Source: CAD feature listing. Evaluate the final solid. Frame: model axes, mm. A direction names the side the tool comes from. Give positions to 0.01 mm unless a question says otherwise; leave off trailing zeros. Loops run counter-clockwise (first coordinate to the right, second up) from the corner with the lowest first, then second, coordinate; pieces in that order, holes last.
from build123d import *

# Parameters (mm, degrees)
SKETCH_W        = 160
SKETCH_H        = 80
PAD_DEPTH       = 32
POCKET_DEPTH    = 26
SKETCH002_R     = 6
POCKET001_DEPTH = 1
SKETCH003_R     = 6
POCKET002_DEPTH = 1
SKETCH004_R     = 3.1
POCKET003_DEPTH = 4
SKETCH005_R     = 3.1
POCKET004_DEPTH = 4
FILLET_R        = 4
FILLET001_R     = 1


with BuildPart() as part:
    # Sketch → Pad (new body)
    with BuildSketch(Plane.XY):
        with Locations((80, 40)):
            Rectangle(SKETCH_W, SKETCH_H)
    extrude(amount=PAD_DEPTH)

    # Sketch001 (on Face6 of Pad) → Pocket (cut)
    with BuildSketch(Plane.XY.offset(32)):
        Polygon((8, 76), (4, 72), (4, 8), (8, 4), (152, 4), (156, 8), (156, 72), (152, 76), align=None)
    extrude(amount=-POCKET_DEPTH, mode=Mode.SUBTRACT)

    # Sketch002 (on Face7 of Pocket) → Pocket001 (cut)
    with BuildSketch(Plane.YZ.offset(4)):
        with Locations((20, 22)):
            Circle(SKETCH002_R)
        with Locations((60, 22)):
            Circle(SKETCH002_R)
    extrude(amount=-POCKET001_DEPTH, mode=Mode.SUBTRACT)

    # Sketch003 (on Face11 of Pocket001) → Pocket002 (cut)
    with BuildSketch(Plane(origin=(156, 0, 0), x_dir=(0, -1, 0), z_dir=(-1, 0, 0))):
        with Locations((-20, 22)):
            Circle(SKETCH003_R)
        with Locations((-60, 22)):
            Circle(SKETCH003_R)
    extrude(amount=-POCKET002_DEPTH, mode=Mode.SUBTRACT)

    # Sketch004 (on Face3 of Pocket002) → Pocket003 (cut)
    with BuildSketch(Plane.YZ.offset(160)):
        with Locations((20, 22)):
            Circle(SKETCH004_R)
        with Locations((60, 22)):
            Circle(SKETCH004_R)
    extrude(amount=-POCKET003_DEPTH, mode=Mode.SUBTRACT)

    # Sketch005 (on Face2 of Pocket003) → Pocket004 (cut)
    with BuildSketch(Plane(origin=(0, 0, 0), x_dir=(0, -1, 0), z_dir=(-1, 0, 0))):
        with Locations((-60, 22)):
            Circle(SKETCH005_R)
        with Locations((-20, 22)):
            Circle(SKETCH005_R)
    extrude(amount=-POCKET004_DEPTH, mode=Mode.SUBTRACT)

    # Fillet
    fillet_edges = [part.edges().sort_by_distance(p)[0] for p in [
        (160, 80, 16),
        (0, 80, 16),
        (0, 0, 16),
        (160, 0, 16),
    ]]
    fillet(fillet_edges, radius=FILLET_R)

    # Fillet001
    fillet001_edges = [part.edges().sort_by_distance(p)[0] for p in [
        (1.171573, 78.828427, 0),
        (0, 40, 0),
        (80, 80, 0),
        (1.171573, 1.171573, 0),
        (80, 0, 0),
        (158.828427, 1.171573, 0),
        (160, 40, 0),
        (158.828427, 78.828427, 0),
    ]]
    fillet(fillet001_edges, radius=FILLET001_R)


solid = part.part
1) Ray query, probe 1 along Y at (x, z) = (107, 30); probe 2 along X at (y, z) = (8, 19); probe 3 along Z at (x, y) = (0.9, 20). Return the intervals inside material, ascending.
Checks:
probe 1: y = 0 to 4, 76 to 80
probe 2: x = 0 to 4, 156 to 160
probe 3: z = 0.01 to 18.9, 25.1 to 32
2) Cut plane A-A (z = 12.5). Return loops of the section in (x, y).
Checks:
outline: (0, 4) arc R4 ccw to (4, 0) - (156, 0) arc R4 ccw to (160, 4) - (160, 76) arc R4 ccw to (156, 80) - (4, 80) arc R4 ccw to (0, 76) - close; hole (4, 8) - (8, 4) - (152, 4) - (156, 8) - (156, 72) - (152, 76) - (8, 76) - (4, 72) - close
3) Cut plane C-C (x = 59). Return loops of the section in (y, z).
Checks:
outline: (0, 1) arc R1 ccw to (1, 0) - (79, 0) arc R1 ccw to (80, 1) - (80, 32) - (76, 32) - (76, 6) - (4, 6) - (4, 32) - (0, 32) - close
4) Reachability of faces 4 (the cylindrical face through (1.141, 1.203, 16.717)), 5 (the flat face through (4, 40, 19)), 6 (the cylindrical face through (156.49, 24.76, 18.35)) from +Z, -Z, +X, -X, +Y, -Y: full face, straight path, thin tool, end or side. Return the list, or none.
Checks:
face 4: +Z, -Z, -X, -Y
face 5: +Z
face 6: none
5) Cut plane D-D (y = 51). Return loops of the section in (x, z), and give its area (3 significant figures).
Checks:
outline: (0, 1) arc R1 ccw to (1, 0) - (159, 0) arc R1 ccw to (160, 1) - (160, 32) - (156, 32) - (156, 6) - (4, 6) - (4, 32) - (0, 32) - close
area: 1,170 mm2
6) Cut plane B-B (y = 60). Return loops of the section in (x, z), and give its area (3 significant figures).
Checks:
outline: (0, 1) arc R1 ccw to (1, 0) - (159, 0) arc R1 ccw to (160, 1) - (160, 18.9) - (157, 18.9) - (157, 16) - (156, 16) - (156, 6) - (4, 6) - (4, 16) - (3, 16) - (3, 18.9) - (0, 18.9) - close; (0, 25.1) - (3, 25.1) - (3, 28) - (4, 28) - (4, 32) - (0, 32) - close; (156, 28) - (157, 28) - (157, 25.1) - (160, 25.1) - (160, 32) - (156, 32) - close
area: 1,110 mm2
7) Contact query for flat-ended pins moving along their axis: P1, Ø7, axis at y = 60, z = 22, coming from the +X side; P2, Ø3.5, axis at y = 20, z = 22, coming from the +X side; P3, Ø6, axis at x = 42, y = 48.5, coming from the +Z side. Output: stop coordinate, or through.
Checks:
P1: stops at x = 160
P2: passes through
P3: stops at z = 6
8) Pull-direction query (X, two-part tool) for faces 1 (the flat face through (156, 40, 19)), 2 (the flat face through (0, 39, 16)), 3 (the flat face through (74, 2, 32)); classes: released by +X, released by -X, zero draft, split by the parting line, or undercut.
Checks:
face 1: undercut
face 2: released by -X
face 3: zero draft
